Autodesk Inventor part; units mm, degrees
ref_plane "YZ Plane" through (0, 0, 0) normal (1, 0, 0) x (0, 1, 0)
ref_plane "XZ Plane" through (0, 0, 0) normal (0, 1, 0) x (-1, 0, 0)
ref_plane "XY Plane" through (0, 0, 0) normal (0, 0, 1) x (1, 0, 0)
sketch "Sketch1" plane through (0, 0, 0) normal (0, 0, 1) x (1, 0, 0)
  line L0 (1.7678, -1.7678) -> (3.9962, 0.4607)
  arc A0 (0, -2.5) -> (1.7678, -1.7678) centre (0, 0) ccw
  line L1 (-3.0076, -2.5) -> (0, -2.5)
  arc A1 (-4.7754, -1.7678) -> (-3.0076, -2.5) centre (-3.0076, 0) ccw
  line L2 (-7.0038, 0.4607) -> (-4.7754, -1.7678)
  line L3 (-7.0038, 2.4) -> (-7.0038, 0.4607)
  line L4 (-5.0038, 2.4) -> (-7.0038, 2.4)
  arc A2 (-5.0038, 2.4) -> (-4.6038, 2.8) centre (-5.0038, 2.8) ccw
  line L5 (-5.7038, 3.9) -> (-4.6038, 2.8)
  line L6 (-11.1038, 3.9) -> (-5.7038, 3.9)
  arc A3 (-11.1038, 3.9) -> (-11.5038, 3.5) centre (-11.1038, 3.5) ccw
  line L7 (-11.5038, -1.9) -> (-11.5038, 3.5)
  line L8 (-10.4038, -3) -> (-11.5038, -1.9)
  arc A4 (-10.4038, -3) -> (-10.0038, -2.6) centre (-10.4038, -2.6) ccw
  line L9 (-10.0038, -0.6) -> (-10.0038, -2.6)
  line L10 (-8.0645, -0.6) -> (-10.0038, -0.6)
  line L11 (-5.836, -2.8284) -> (-8.0645, -0.6)
  arc A5 (-5.1038, -4.5962) -> (-5.836, -2.8284) centre (-7.6038, -4.5962) ccw
  line L12 (-5.1038, -7.6038) -> (-5.1038, -4.5962)
  arc A6 (-5.836, -9.3716) -> (-5.1038, -7.6038) centre (-7.6038, -7.6038) ccw
  line L13 (-8.0645, -11.6) -> (-5.836, -9.3716)
  line L14 (-10.0038, -11.6) -> (-8.0645, -11.6)
  line L15 (-10.0038, -9.6) -> (-10.0038, -11.6)
  arc A7 (-10.0038, -9.6) -> (-10.4038, -9.2) centre (-10.4038, -9.6) ccw
  line L16 (-11.5038, -10.3) -> (-10.4038, -9.2)
  line L17 (-11.5038, -15.7) -> (-11.5038, -10.3)
  arc A8 (-11.5038, -15.7) -> (-11.1038, -16.1) centre (-11.1038, -15.7) ccw
  line L18 (-5.7038, -16.1) -> (-11.1038, -16.1)
  line L19 (-4.6038, -15) -> (-5.7038, -16.1)
  arc A9 (-4.6038, -15) -> (-5.0038, -14.6) centre (-5.0038, -15) ccw
  line L20 (-7.0038, -14.6) -> (-5.0038, -14.6)
  line L21 (-7.0038, -12.6607) -> (-7.0038, -14.6)
  line L22 (-4.7754, -10.4322) -> (-7.0038, -12.6607)
  arc A10 (-3.0076, -9.7) -> (-4.7754, -10.4322) centre (-3.0076, -12.2) ccw
  line L23 (0, -9.7) -> (-3.0076, -9.7)
  arc A11 (1.7678, -10.4322) -> (0, -9.7) centre (0, -12.2) ccw
  line L24 (3.9962, -12.6607) -> (1.7678, -10.4322)
  line L25 (3.9962, -14.6) -> (3.9962, -12.6607)
  line L26 (1.9962, -14.6) -> (3.9962, -14.6)
  arc A12 (1.9962, -14.6) -> (1.5962, -15) centre (1.9962, -15) ccw
  line L27 (2.6962, -16.1) -> (1.5962, -15)
  line L28 (8.0962, -16.1) -> (2.6962, -16.1)
  arc A13 (8.0962, -16.1) -> (8.4962, -15.7) centre (8.0962, -15.7) ccw
  line L29 (8.4962, -10.3) -> (8.4962, -15.7)
  line L30 (7.3962, -9.2) -> (8.4962, -10.3)
  arc A14 (7.3962, -9.2) -> (6.9962, -9.6) centre (7.3962, -9.6) ccw
  line L31 (6.9962, -11.6) -> (6.9962, -9.6)
  line L32 (5.0569, -11.6) -> (6.9962, -11.6)
  line L33 (2.8284, -9.3716) -> (5.0569, -11.6)
  arc A15 (2.0962, -7.6038) -> (2.8284, -9.3716) centre (4.5962, -7.6038) ccw
  line L34 (2.0962, -4.5962) -> (2.0962, -7.6038)
  arc A16 (2.8284, -2.8284) -> (2.0962, -4.5962) centre (4.5962, -4.5962) ccw
  line L35 (5.0569, -0.6) -> (2.8284, -2.8284)
  line L36 (6.9962, -0.6) -> (5.0569, -0.6)
  line L37 (6.9962, -2.6) -> (6.9962, -0.6)
  arc A17 (6.9962, -2.6) -> (7.3962, -3) centre (7.3962, -2.6) ccw
  line L38 (8.4962, -1.9) -> (7.3962, -3)
  line L39 (8.4962, 3.5) -> (8.4962, -1.9)
  arc A18 (8.4962, 3.5) -> (8.0962, 3.9) centre (8.0962, 3.5) ccw
  line L40 (2.6962, 3.9) -> (8.0962, 3.9)
  line L41 (1.5962, 2.8) -> (2.6962, 3.9)
  arc A19 (1.5962, 2.8) -> (1.9962, 2.4) centre (1.9962, 2.8) ccw
  line L42 (3.9962, 2.4) -> (1.9962, 2.4)
  line L43 (3.9962, 0.4607) -> (3.9962, 2.4)
  circle A20 centre (-1.5038, -6.1) radius 2.5
  point P0 (0, 0)
extrude "Extrusion1" add sketch "Sketch1" along normal blind 250
ref_plane "Work Plane1" through (-1.5038, -15.7, 0) normal (-1, 0, 0) x (0, 0, 1)
properties part number "00_VSlot_20mm_200"
Here's how the part is built. I have some questions about the finished solid (model axes, mm). Round coordinates to 2 decimals unless told otherwise and drop trailing zeros. Answer as CSV lines item,"result".
1. If I drill on L1, parallel to Y at x = -1.5, z = 15; L2, parallel to Y at x = -9.5, z = 74.5; L3, parallel to X at y = -11, z = 167, over which ranges is the centre line in solid material (lowest first)?
Final values:
L1,"y = -9.7 to -8.6, -3.6 to -2.5"
L2,"y = -16.1 to -11.6, -0.6 to 3.9"
L3,"x = -11.5 to -10, -7.46 to -5.34, 2.34 to 4.46, 7 to 8.5"
2. Thinking about a two-plate mould opening in X: for faces 1 (the face through (-11.504, -13, 123)), 2 (the face through (5, -16.1, 123)), 3 (the face through (-1.83, -8.58, 123.25)), which applies, released by +X, released by -X, zero draft, split by the parting line, or undercut?
Final values:
face 1,"released by -X"
face 2,"zero draft"
face 3,"undercut"
3. For pin 1 (2.5 mm diameter, centred on y = -5.5, z = 156.5, fed in from -X); pin 2 (2.5 mm diameter, centred on x = -1, z = 139.5, fed in from -Y), each with a flat end and sliding along its axis, tell me the tip position at first contact or that it passes through.
Final values:
pin 1,"stops at x = -5.13"
pin 2,"stops at y = -9.71"
